```python
from build123d import *

# Parameters (mm, degrees)
SKETCH1_W           = 5
SKETCH1_H           = 60
BOSS_EXTRUDE1_DEPTH = 5
SKETCH2_W           = 5
SKETCH2_H           = 60
BOSS_EXTRUDE2_DEPTH = 20
SKETCH3_R           = 2.5
BOSS_EXTRUDE3_DEPTH = 20
SKETCH4_W           = 5
SKETCH4_H           = 60
BOSS_EXTRUDE4_DEPTH = 22
SKETCH5_R           = 4.1
SKETCH5_R_2         = 1.75
CUT_EXTRUDE1_DEPTH  = 6


with BuildPart() as part:
    # Sketch1 → Boss-Extrude1 (new body)
    with BuildSketch(Plane(origin=(0, 0, 0), x_dir=(0, 0, -1), z_dir=(1, 0, 0))):
        with Locations((10.587248322, 7.600671141)):
            Rectangle(SKETCH1_W, SKETCH1_H)
    extrude(amount=BOSS_EXTRUDE1_DEPTH)

    # Sketch2 → Boss-Extrude2 (add)
    with BuildSketch(Plane(origin=(5, 0, 0), x_dir=(0, 0, -1), z_dir=(1, 0, 0))):
        with Locations((10.587248322, 7.600671141)):
            Rectangle(SKETCH2_W, SKETCH2_H)
    extrude(amount=BOSS_EXTRUDE2_DEPTH)

    # Sketch3 → Boss-Extrude3 (add)
    with BuildSketch(Plane(origin=(0, 0, -13.087248322), x_dir=(-1, 0, 0), z_dir=(0, 0, -1))):
        with Locations((-17.5, 7.600671141)):
            Circle(SKETCH3_R)
    extrude(amount=BOSS_EXTRUDE3_DEPTH)

    # Sketch4 → Boss-Extrude4 (add)
    with BuildSketch(Plane.ZY):
        with Locations((-10.587248322, 7.600671141)):
            Rectangle(SKETCH4_W, SKETCH4_H)
    extrude(amount=BOSS_EXTRUDE4_DEPTH)

    # Sketch5 → Cut-Extrude1 (cut, through all)
    with BuildSketch(Plane(origin=(0, 0, -13.087248322), x_dir=(-1, 0, 0), z_dir=(0, 0, -1))):
        with Locations((13, 28.600671141)):
            Circle(SKETCH5_R)
        with Locations((13, -13.399328859)):
            Circle(SKETCH5_R)
        with Locations((13, -1.399328859)):
            Circle(SKETCH5_R_2)
        with Locations((13, 16.600671141)):
            Circle(SKETCH5_R_2)
    extrude(amount=-CUT_EXTRUDE1_DEPTH, mode=Mode.SUBTRACT)


solid = part.part
```
CAD build for the part. Positions are in the model's coordinates, mm. Coordinates: 2 decimals unless noted, no trailing zeros. Order: outer loops, then holes, each group sorted by start corner. A loop starts at its lowest first (then second) coordinate and runs counter-clockwise, first axis right, second up. Notation, with made-up numbers: M 8.5,-9.75 L 24.5,-9.75 A18 ccw 24.5,16.25 Z; hole C 10,42 d3. An arc over 180 degrees is marked long. Answer as CSV lines item,"result".
1) Flat gauge pins, fed straight in: P1, Ø3, axis at x = -1, z = -14, coming from the +Y side; P2, Ø4, axis at x = -13, y = -1.4, coming from the -Z side; P3, Ø2, axis at x = 19, z = -23, coming from the -Y side. Where does each tip first touch, or does it go through?
Verdict:
P1,"y = 37.6"
P2,"z = -13.09"
P3,"y = 5.15"
2) Cut at B-B (y = 26). List the corners of the cut face in (x, z), then the cut area to 3 significant figures.
Verdict:
outline,"M -22,-13.09 L -16.17,-13.09 L -16.17,-8.09 L -22,-8.09 Z; M -9.83,-13.09 L 25,-13.09 L 25,-8.09 L -9.83,-8.09 Z"
area,"203 mm2"
3) Cut at A-A (x = -13). List the corners of the cut face in (y, z).
Verdict:
outline,"M -22.4,-13.09 L -17.5,-13.09 L -17.5,-8.09 L -22.4,-8.09 Z; M -9.3,-13.09 L -3.15,-13.09 L -3.15,-8.09 L -9.3,-8.09 Z; M 0.35,-13.09 L 14.85,-13.09 L 14.85,-8.09 L 0.35,-8.09 Z; M 18.35,-13.09 L 24.5,-13.09 L 24.5,-8.09 L 18.35,-8.09 Z; M 32.7,-13.09 L 37.6,-13.09 L 37.6,-8.09 L 32.7,-8.09 Z"
4) Cut at C-C (z = -11). List the corners of the cut face in (x, y), then the cut area to 3 significant figures.
Verdict:
outline,"M -22,-22.4 L 25,-22.4 L 25,37.6 L -22,37.6 Z; hole C -13,-13.4 d8.2; hole C -13,28.6 d8.2; hole C -13,-1.4 d3.5; hole C -13,16.6 d3.5"
area,"2,700 mm2"
5) Drill centre lines: L1, parallel to Y at x = -13, z = -9.85; L2, parallel to Z at x = 21.5, y = -0.5; L3, parallel to X at y = 5.5, z = -24.25. Where is each one in solid material? Low to high. Write a range as from..to.
Verdict:
L1,"-22.4..-17.5, -9.3..-3.15, 0.35..14.85, 18.35..24.5, 32.7..37.6"
L2,"-13.09..-8.09"
L3,"16.14..18.86"
6) Cut at D-D (x = 17.5). List the corners of the cut face in (y, z), then the cut area to 3 significant figures.
Verdict:
outline,"M -22.4,-13.09 L 5.1,-13.09 L 5.1,-33.09 L 10.1,-33.09 L 10.1,-13.09 L 37.6,-13.09 L 37.6,-8.09 L -22.4,-8.09 Z"
area,"400 mm2"
7) Mould opens along X. For faces 1 (the cylindrical face through (20, 7.7, -22.9)), 2 (the flat face through (-22, 8, -11)), 3 (the cylindrical face through (-14.67, 17.13, -10.62)) say: released by +X, released by -X, zero draft, split by the parting line, or undercut.
Verdict:
face 1,"split by the parting line"
face 2,"released by -X"
face 3,"undercut"
